from build123d import *

# Parameters (mm, degrees)
F0_R     = 12.7
F1_DEPTH = 15.875
F0_R_2   = 16.51
F2_DEPTH = 19.05
F4_DEPTH = 3.175
F5_R     = 2.54
F6_DEPTH = 19.051
F7_R     = 5.08


with BuildPart() as f1:
    # F0 (on Top) → F1 (new body)
    with BuildSketch(Plane.XY):
        Circle(F0_R)
    extrude(amount=F1_DEPTH)

    # F0 (on Top) → F2 (join)
    with BuildSketch(Plane.XY):
        Circle(F0_R_2)
        Circle(F0_R, mode=Mode.SUBTRACT)
    extrude(amount=F2_DEPTH)

    # F3 (on face) → F4 (join, through all)
    with BuildSketch(Plane.XY.offset(15.875)):
        with BuildLine():
            Line((-11.43, -5.535802), (-11.43, 5.535802))
            ThreePointArc((-11.43, 5.535802), (-12.7, 0), (-11.43, -5.535802))
        make_face()
    extrude(amount=F4_DEPTH)

    # F5 (on face) → F6 (cut, through all)
    with BuildSketch(Plane(origin=(0, 0, 0), x_dir=(1, 0, 0), z_dir=(0, 0, -1))):
        Circle(F5_R)
    extrude(amount=-F6_DEPTH, mode=Mode.SUBTRACT)

    # F7
    f7_edges = [f1.edges().sort_by_distance(p)[0] for p in [
        (-16.51, 0, 0),
        (-2.54, 0, 0),
    ]]
    fillet(f7_edges, radius=F7_R)


solid = f1.part
For this review, take the finished solid that the model builds, in its own axes (mm). A direction names the side the tool comes from. Round coordinates to 2 decimals unless told otherwise and drop trailing zeros. Loops run counter-clockwise (first coordinate to the right, second up) from the corner with the lowest first, then second, coordinate; pieces in that order, holes last. Notation, with made-up numbers: (-20.5, -14.75) - (30.5, -14.75) arc R35 cw to (30.5, 18.25) - close; hole circle Ø7 at (-22.5, -6). An arc over 180 degrees is marked (long way). Put each result on its own line as item: value. Start each with the question number.
1. Consider section A-A on y = 0. State the section outline as (x, z) points (3 decimals).
2. Insertion check: P1, Ø2, axis at x = 2, y = 1, coming from the +Z side (3 decimals); P2, Ø1.5, axis at y = -4.5, z = 15.5, coming from the +X side; P3, Ø1, axis at y = 1.5, z = 16.5, coming from the -X side. Each pin has a flat end and moves straight along its axis. Give the tip position at first contact, or say it passes through.
3. For faces 1 (the flat face through (2.4, -7.5, 0)), 2 (the flat face through (-11.43, 0, 17)), list the 3-axis set-ups (+Z, -Z, +X, -X, +Y, -Y) from which the entire face can be reached by the end or side of a thin tool; tool diameter is ignored.
4. Consider section C-C on z = 8.75. State the section outline as (x, y) points, plus the area to 3 significant figures.
5. Consider section B-B on x = 0. State the section outline as (y, z) points (3 decimals).
6. For probe 1 along Y at (x, z) = (0, 13.5); probe 2 along Y at (x, z) = (0, 16.7); probe 3 along Z at (x, y) = (-5, 9) (3 decimals), list the stretches that pass through material, from the lowest coordinate up. Write a range as [from, to].
7. Mouldability with a two-part tool opening along Y and no side actions: class faces 3 (the flat face through (0, -3, 15.875)), 4 (the cylindrical face through (15.748, 4.959, 11.967)), 5 (the flat face through (-12, 1, 19.05)) as +Y half, -Y half, draft (parallel to the pull), parting line (faces both ways), or undercut.
Result sheet:
1. outline: (-16.51, 5.08) arc R5.08 ccw to (-11.43, 0) - (-7.62, 0) arc R5.08 ccw to (-2.54, 5.08) - (-2.54, 15.875) - (-11.43, 15.875) - (-11.43, 19.05) - (-16.51, 19.05) - close; (2.54, 5.08) arc R5.08 ccw to (7.62, 0) - (11.43, 0) arc R5.08 ccw to (16.51, 5.08) - (16.51, 19.05) - (12.7, 19.05) - (12.7, 15.875) - (2.54, 15.875) - close
2. P1: z = 15.875
2. P2: x = 16.08
2. P3: x = -16.48
3. face 1: -Z, +X, -X, +Y, -Y
3. face 2: +Z
4. outline: circle Ø33.02 at (0, 0); hole circle Ø5.08 at (0, 0)
4. area: 836 mm^2
5. outline: (-16.51, 5.08) arc R5.08 ccw to (-11.43, 0) - (-7.62, 0) arc R5.08 ccw to (-2.54, 5.08) - (-2.54, 15.875) - (-12.7, 15.875) - (-12.7, 19.05) - (-16.51, 19.05) - close; (2.54, 5.08) arc R5.08 ccw to (7.62, 0) - (11.43, 0) arc R5.08 ccw to (16.51, 5.08) - (16.51, 19.05) - (12.7, 19.05) - (12.7, 15.875) - (2.54, 15.875) - close
6. probe 1: [-16.51, -2.54], [2.54, 16.51]
6. probe 2: [-16.51, -12.7], [12.7, 16.51]
6. probe 3: [0, 15.875]
7. face 3: undercut
7. face 4: parting line
7. face 5: draft
